Here's the drawing with two shaded views (mm, measured from the low corner). I have some questions. A direction names the side the tool comes from. Give positions to 0.01 mm unless a question says otherwise; leave off trailing zeros. Loops run counter-clockwise (first coordinate to the right, second up) from the corner with the lowest first, then second, coordinate; pieces in that order, holes last. Notation, with made-up numbers: M -34,86.5 L -23,86.5 A12 cw -23,94.5 Z; hole C 67,60 d6. An arc over 180 degrees is marked long. Answer in a Markdown table with one row per item. Add a question column.
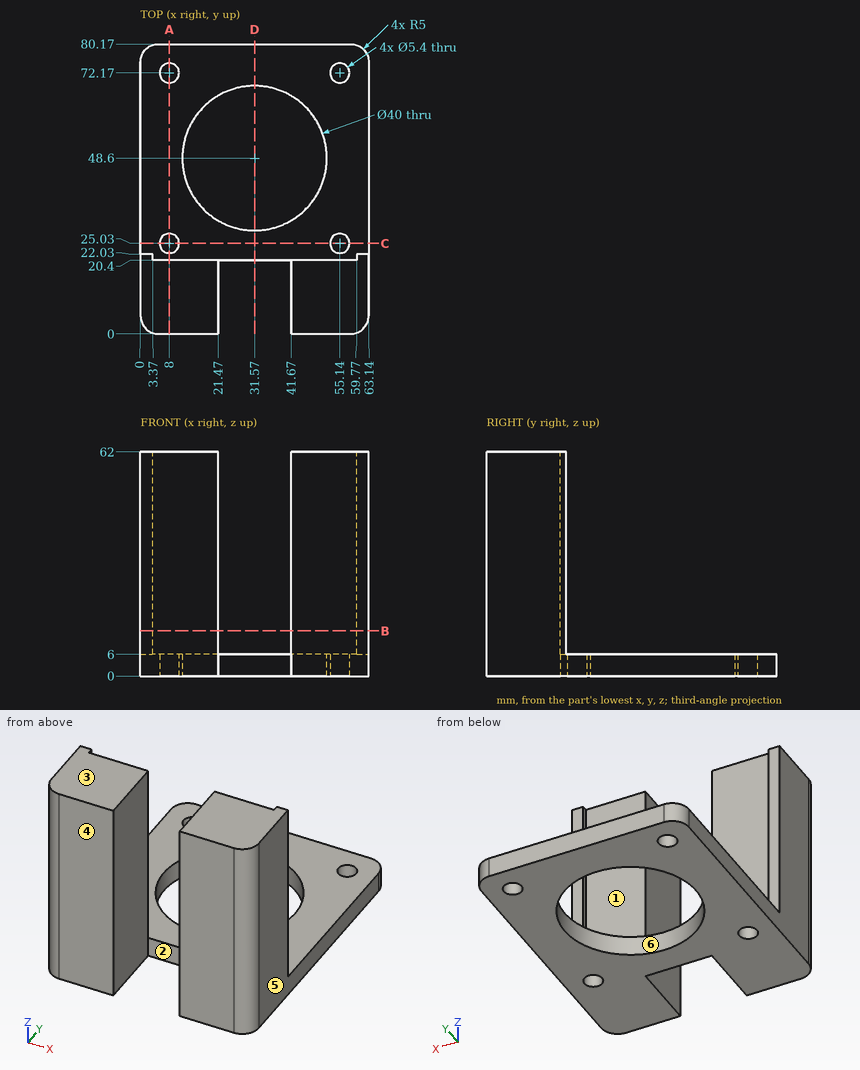
Item 1: Suppose I cut it at D-D (x = 31.57). List the corners of the cut face in (y, z) for me, then the cut area to 3 significant figures.
Item 2: For P1, Ø5, axis at x = 32, z = 3.5, coming from the -Y side; P2, Ø1.7, axis at x = 61.5, z = 26.5, coming from the +Y side; P3, Ø8, axis at x = 48.5, y = 62.5, coming from the +Z side, each with a flat end and sliding along its axis, tell me the tip position at first contact or that it passes through.
Item 3: Suppose I cut it at A-A (x = 8). List the corners of the cut face in (y, z) for me.
Item 4: For the marked faces 1, 2 and 3, which set-ups out of +Z, -Z, +X, -X, +Y, -Y let a thin tool reach every point of the face, with its end or its side?
Item 5: If we mould it in two halves opening along X, with no side actions, what happens to the marked faces 4, 5 and 6? For each: +X half, -X half, draft (parallel to the pull), parting line (faces both ways), or undercut.
Item 6: Suppose I cut it at B-B (z = 12.5). List the corners of the cut face in (x, y) for me, then the cut area to 3 significant figures.
Item 7: I need wall thicknesses on L1, parallel to Y at x = 8, z = 1.4; L2, parallel to X at y = 7.5, z = 44; L3, parallel to Y at x = 31.57, z = 2.45. Which ranges of each line are inside material? Lowest first, please.
Item 8: Suppose I cut it at C-C (y = 25.03). List the corners of the cut face in (x, z) for me.
Values found:
| question | item | result |
|---|---|---|
| 1 | outline | M 20.4,0 L 28.6,0 L 28.6,6 L 20.4,6 Z; M 68.6,0 L 80.17,0 L 80.17,6 L 68.6,6 Z |
| 1 | area | 119 mm² |
| 2 | P1 | y = 20.4 |
| 2 | P2 | y = 22.03 |
| 2 | P3 | z = 6 |
| 3 | outline | M 0,0 L 22.33,0 L 22.33,6 L 20.4,6 L 20.4,62 L 0,62 Z; M 27.73,0 L 69.47,0 L 69.47,6 L 27.73,6 Z; M 74.87,0 L 80.17,0 L 80.17,6 L 74.87,6 Z |
| 4 | face 1 | +Z, +Y |
| 4 | face 2 | +Z, -Z, -Y |
| 4 | face 3 | +Z, +X, -X, +Y, -Y |
| 5 | face 4 | draft |
| 5 | face 5 | +X half |
| 5 | face 6 | undercut |
| 6 | outline | M 0,5 A5 ccw 5,0 L 21.47,0 L 21.47,20.4 L 3.37,20.4 L 3.37,22.03 L 0,22.03 Z; M 41.67,0 L 58.14,0 A5 ccw 63.14,5 L 63.14,22.03 L 59.77,22.03 L 59.77,20.4 L 41.67,20.4 Z |
| 6 | area | 876 mm² |
| 7 | L1 | 0 to 22.33, 27.73 to 69.47, 74.87 to 80.17 |
| 7 | L2 | 0 to 21.47, 41.67 to 63.14 |
| 7 | L3 | 20.4 to 28.6, 68.6 to 80.17 |
| 8 | outline | M 0,0 L 5.3,0 L 5.3,6 L 0,6 Z; M 10.7,0 L 52.44,0 L 52.44,6 L 10.7,6 Z; M 57.84,0 L 63.14,0 L 63.14,6 L 57.84,6 Z |
